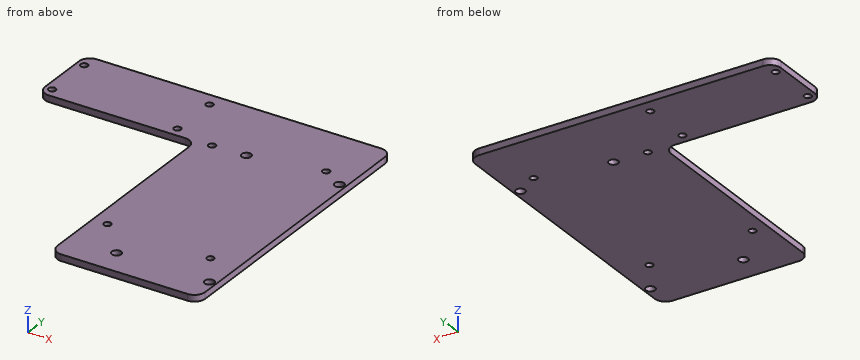
from build123d import *

# Parameters (mm, degrees)
F1_DEPTH = 3
F2_D     = 3.3
F3_D     = 4.3
F4_R     = 5


# Not quite as in the source:
# - a feature names something its author has since deleted; it is built from what else it names


with BuildPart() as f1:
    # F0 (on Top) → F1 (new body)
    with BuildSketch(Plane.XY):
        Polygon((-43.9476147294, -59.139739722), (24.4538411498, -59.139739722), (24.4538411498, 79.5589722693), (-117.0655786991, 79.5589722693), (-117.0655786991, 45.1967306435), (-43.9476147294, 45.1967306435), align=None)
    extrude(amount=F1_DEPTH)

    # F2 (through all)
    with Locations(Plane(origin=(0, 0, 0), x_dir=(1, 0, 0), z_dir=(0, 0, -1))):
        with Locations((-113.6049106717, -72.9293674231), (-113.6049106717, -49.9293674231), (-55.6049106717, -49.9293674231), (-55.6049106717, -72.9293674231), (-37.0104938323, -45.9071589798), (11.4895061677, -52.6071589798), (11.4895061677, 30.2928410202), (-37.0104938323, 28.9928410202)):
            Hole(F2_D / 2)

    # F3 (through all)
    with Locations(Plane(origin=(0, 0, 0), x_dir=(1, 0, 0), z_dir=(0, 0, -1))):
        with Locations((-21.5, -46.5), (21.5, -46.5), (21.5, 46.5), (-21.5, 46.5)):
            Hole(F3_D / 2)

    # F4
    f4_edges = [f1.edges().sort_by_distance(p)[0] for p in [
        (-117.065579, 79.558972, 1.5),
        (-43.947615, 45.196731, 1.5),
        (-117.065579, 45.196731, 1.5),
        (24.453841, 79.558972, 1.5),
        (24.453841, -59.13974, 1.5),
        (-43.947615, -59.13974, 1.5),
    ]]
    fillet(f4_edges, radius=F4_R)


solid = f1.part
Verification items for the finished model (mm, model axes). Coordinates: 2 decimals unless noted, no trailing zeros. Write each loop counter-clockwise with the first axis right and the second up, starting at its lowest first coordinate (ties: lowest second). Pieces come first, ordered by that corner, then holes. Notation, with made-up numbers: M 53.5,41 L 95.5,41 A6 ccw 95.5,51 Z; hole C -5,8.5 d2. An arc over 180 degrees is marked long. Use a Markdown table: item, result.
Q1. Thickness scan on line 1 (X direction, y = -46.5, z = 2.4); line 2 (Y direction, x = -21.5, z = 2.25); line 3 (X direction, y = 72, z = 1.9). Record the ranges inside material, lowest first.
Reply:
| item | result |
|---|---|
| line 1 | x = -43.95 to -23.65, -19.35 to 19.35, 23.65 to 24.45 |
| line 2 | y = -59.14 to -48.65, -44.35 to 44.35, 48.65 to 79.56 |
| line 3 | x = -117.07 to -114.97, -112.24 to -56.97, -54.24 to 24.45 |
Q2. Sectioned sample at A-A, the plane x = -21.5. Record the boundary of the cut face in (y, z).
Reply:
| item | result |
|---|---|
| outline | M -59.14,0 L -48.65,0 L -48.65,3 L -59.14,3 Z; M -44.35,0 L 44.35,0 L 44.35,3 L -44.35,3 Z; M 48.65,0 L 79.56,0 L 79.56,3 L 48.65,3 Z |
Q3. Sectioned sample at C-C, the plane z = 2.55. Count the separate pieces of the cut face and the enclosed holes in it, plus the area to 3 significant figures.
Reply:
| item | result |
|---|---|
| separate pieces | 1 |
| enclosed holes | 12 |
| area | 11,900 mm² |
Q4. Sectioned sample at B-B, the plane y = -46.5. Record the boundary of the cut face in (x, z).
Reply:
| item | result |
|---|---|
| outline | M -43.95,0 L -23.65,0 L -23.65,3 L -43.95,3 Z; M -19.35,0 L 19.35,0 L 19.35,3 L -19.35,3 Z; M 23.65,0 L 24.45,0 L 24.45,3 L 23.65,3 Z |
Q5. Sectioned sample at D-D, the plane x = -66. Record the boundary of the cut face in (y, z).
Reply:
| item | result |
|---|---|
| outline | M 45.2,0 L 79.56,0 L 79.56,3 L 45.2,3 Z |
Q6. Go/stop test with flat-tipped pins: P1, Ø1.5, axis at x = -73, z = 1.5, coming from the -Y side; P2, Ø4.5, axis at x = -55.6, y = 49.93, coming from the -Z side; P3, Ø1.5, axis at y = -22.5, z = 2, coming from the -X side. Record where each tip stops, or that it passes through.
Reply:
| item | result |
|---|---|
| P1 | stops at y = 45.2 |
| P2 | stops at z = 0 |
| P3 | stops at x = -43.95 |
